from build123d import *

# Parameters (mm, degrees)
EXTRUDE1_DEPTH                 = 200
FILLET1_R                      = 0.25
F_3_5_3_5_DIAMETER_HOLE1_D     = 3.5
F_4_5_4_5_DIAMETER_HOLE1_D     = 4.5
F_4_5_4_5_DIAMETER_HOLE1_DEPTH = 1
F_4_5_4_5_DIAMETER_HOLE1_TIP   = 1.351936393
LPATTERN1_COUNT                = 4
LPATTERN1_PITCH                = 38.4


with BuildPart() as part:
    # Sketch1 → Extrude1 (new body)
    with BuildSketch(Plane.XY):
        Polygon((0, 0), (0, 24), (-12, 24), (-12, 25), (13, 25), (13, 24), (1, 24), (1, 0), align=None)
    extrude(amount=EXTRUDE1_DEPTH)

    # Fillet1
    fillet1_edges = [part.edges().sort_by_distance(p)[0] for p in [
        (0, 0, 100),
        (-12, 24, 100),
        (-12, 25, 100),
        (13, 24.5, 200),
        (13, 25, 100),
        (13, 24, 100),
        (1, 0, 100),
        (-12, 24.5, 200),
        (0.5, 0, 200),
        (-12, 24.5, 0),
        (13, 24.5, 0),
        (0.5, 0, 0),
    ]]
    fillet(fillet1_edges, radius=FILLET1_R)

    # Ø3.5 (3.5) Diameter Hole1 (through all)
    with Locations(Plane(origin=(-6, 24, 196), x_dir=(-1, 0, 0), z_dir=(0, -1, 0))):
        with Locations((0, 0), (-13, 0), (0, 192), (-13, 192)):
            Hole(F_3_5_3_5_DIAMETER_HOLE1_D / 2)

    # Ø4.5 (4.5) Diameter Hole1
    with Locations(Plane(origin=(-5, 25, 176), x_dir=(0, 0, 1), z_dir=(0, 1, 0))):
        with Locations((0, 0), (-76, 0)):
            Hole(F_4_5_4_5_DIAMETER_HOLE1_D / 2, depth=F_4_5_4_5_DIAMETER_HOLE1_DEPTH)
            with Locations((0, 0, -(F_4_5_4_5_DIAMETER_HOLE1_DEPTH + F_4_5_4_5_DIAMETER_HOLE1_TIP / 2))):  # 118° drill point
                Cone(0, F_4_5_4_5_DIAMETER_HOLE1_D / 2, F_4_5_4_5_DIAMETER_HOLE1_TIP, mode=Mode.SUBTRACT)

    # Sketch10 → Ø4.5 (4.5) Diameter Hole2 (revolve, cut)
    with BuildSketch(Plane(origin=(7, 24, 157.6), x_dir=(0, 0, -1), z_dir=(1, 0, 0))):
        Polygon((0, 0), (0, 2.351936393), (2.25, 1), (2.25, 0), align=None)
    f_4_5_4_5_diameter_hole2 = revolve(axis=Axis((7, 17.65, 157.6), (0, 1, 0)), mode=Mode.SUBTRACT)

    # LPattern1: Ø4.5 (4.5) Diameter Hole2 ×4
    with Locations(*[(0, 0, -i * LPATTERN1_PITCH) for i in range(1, LPATTERN1_COUNT)]):
        add(f_4_5_4_5_diameter_hole2, mode=Mode.SUBTRACT)


solid = part.part
Geometry check sheet. Reference: the model listing, model coordinates, mm. A direction names the side the tool comes from. Give positions to 0.01 mm unless a question says otherwise; leave off trailing zeros. Order: outer loops, then holes, each group sorted by start corner. A loop starts at its lowest first (then second) coordinate and runs counter-clockwise, first axis right, second up.
1. Depth check by flat-ended pin: pin 1 (2 mm diameter, centred on x = -6, z = 4, fed in from +Y); pin 2 (5.5 mm diameter, centred on x = -6, z = 196, fed in from -Y); pin 3 (7 mm diameter, centred on y = 16, z = 140.5, fed in from +X); pin 4 (5 mm diameter, centred on y = 7.5, z = 73.5, fed in from -X). Enter the tip coordinate at first touch or a pass-through.
Completed:
pin 1: passes through
pin 2: stops at y = 24
pin 3: stops at x = 1
pin 4: stops at x = 0
2. Sectioned sample at D-D (z = 55.5). Record the boundary of the cut face in (x, y), then the cut area to 3 significant figures.
Completed:
outline: (-12, 24.25) arc R0.25 ccw to (-11.75, 24) - (0, 24) - (0, 0.25) arc R0.25 ccw to (0.25, 0) - (0.75, 0) arc R0.25 ccw to (1, 0.25) - (1, 24) - (12.75, 24) arc R0.25 ccw to (13, 24.25) - (13, 24.75) arc R0.25 ccw to (12.75, 25) - (-11.75, 25) arc R0.25 ccw to (-12, 24.75) - close
area: 48.9 mm2
3. Scan lines: line 1 (X direction, y = 24.75, z = 4); line 2 (X direction, y = 24.75, z = 157.6); line 3 (Z direction, x = -5, y = 24.6). Record each from-to range of solid material in increasing order.
Completed:
line 1: x = -12 to -7.75, -4.25 to 5.25, 8.75 to 13
line 2: x = -12 to 4.75, 9.25 to 13
line 3: z = 0 to 2.56, 5.44 to 97.75, 102.25 to 173.75, 178.25 to 194.56, 197.44 to 200
4. Sectioned sample at A-A (z = 80.8). Record the boundary of the cut face in (x, y), then the cut area to 3 significant figures.
Completed:
outline: (-12, 24.25) arc R0.25 ccw to (-11.75, 24) - (0, 24) - (0, 0.25) arc R0.25 ccw to (0.25, 0) - (0.75, 0) arc R0.25 ccw to (1, 0.25) - (1, 24) - (4.75, 24) - (4.75, 25) - (-11.75, 25) arc R0.25 ccw to (-12, 24.75) - close; (9.25, 24) - (12.75, 24) arc R0.25 ccw to (13, 24.25) - (13, 24.75) arc R0.25 ccw to (12.75, 25) - (9.25, 25) - close
area: 44.4 mm2
5. Access from +Z, -Z, +X, -X, +Y, -Y to the whole of each face (thin tool, end or side, straight path). Record for faces 1 (the face through (-5.86, 24.49, 97.92)), 2 (the face through (0, 12, 99)), 3 (the face through (1, 12, 99)).
Completed:
face 1: +Y, -Y
face 2: +Z, -Z, -X, -Y
face 3: +Z, -Z, +X, -Y
6. Draft check along Z on faces 4 (the face through (-6.38, 24.51, 197.71)), 5 (the face through (7, 24, 99)), 6 (the face through (0.6, 18.2, 200)). Enter one of: pulls with the +Z half, pulls with the -Z half, needs draft (parallel to the pull), parting line crosses it, or undercut.
Completed:
face 4: undercut
face 5: needs draft
face 6: pulls with the +Z half
7. Sectioned sample at B-B (z = 196). Record the boundary of the cut face in (x, y), then the cut area to 3 significant figures.
Completed:
outline: (-12, 24.25) arc R0.25 ccw to (-11.75, 24) - (-7.75, 24) - (-7.75, 25) - (-11.75, 25) arc R0.25 ccw to (-12, 24.75) - close; (-4.25, 24) - (0, 24) - (0, 0.25) arc R0.25 ccw to (0.25, 0) - (0.75, 0) arc R0.25 ccw to (1, 0.25) - (1, 24) - (5.25, 24) - (5.25, 25) - (-4.25, 25) - close; (8.75, 24) - (12.75, 24) arc R0.25 ccw to (13, 24.25) - (13, 24.75) arc R0.25 ccw to (12.75, 25) - (8.75, 25) - close
area: 41.9 mm2
8. Sectioned sample at C-C (x = 7). Record the boundary of the cut face in (y, z), then the cut area to 3 significant figures.
Completed:
outline: (24, 0) - (25, 0) - (25, 2.25) - (24, 2.25) - close; (24, 5.75) - (25, 5.75) - (25, 40.15) - (24, 40.15) - close; (24, 44.65) - (25, 44.65) - (25, 78.55) - (24, 78.55) - close; (24, 83.05) - (25, 83.05) - (25, 116.95) - (24, 116.95) - close; (24, 121.45) - (25, 121.45) - (25, 155.35) - (24, 155.35) - close; (24, 159.85) - (25, 159.85) - (25, 194.25) - (24, 194.25) - close; (24, 197.75) - (25, 197.75) - (25, 200) - (24, 200) - close
area: 175 mm2
